from build123d import *

# Parameters (mm, degrees)
BOSS_EXTRUDE1_DEPTH = 4
BOSS_EXTRUDE1_DRAFT = 1
SHELL1_T            = -0.5
SKETCH2_R           = 2
BOSS_EXTRUDE2_DEPTH = 5.5
BOSS_EXTRUDE2_TAPER = 1.5
CIRPATTERN1_COUNT   = 4
SKETCH4_R           = 1.605977431
CUT_EXTRUDE1_DEPTH  = 5.5
CUT_EXTRUDE1_DRAFT  = 1.5
RIB2_START          = -8.069744096
RIB2_DEPTH          = 6.232014751
RIB2_START_2        = 1.837729345
RIB2_2_DEPTH        = 6.232014751
RIB2_START_3        = -0.25
RIB2_3_DEPTH        = 0.4999999
RIB2_START_4        = -5.909834066
RIB2_4_DEPTH        = 4.072104721
RIB2_5_DEPTH        = 4.072104621


with BuildPart() as part:
    # Sketch1 → Boss-Extrude1 (with draft: the straight prism first)
    with BuildSketch(Plane(origin=(0, 0, 0), x_dir=(1, 0, 0), z_dir=(0, 1, 0))):
        with BuildLine():
            Line((-7.5, -6.375), (7.5, -6.375))
            ThreePointArc((7.5, -6.375), (8.207106781, -6.082106781), (8.5, -5.375))
            Line((8.5, -5.375), (8.5, 5.375))
            ThreePointArc((8.5, 5.375), (8.207106781, 6.082106781), (7.5, 6.375))
            Line((7.5, 6.375), (-7.5, 6.375))
            ThreePointArc((-7.5, 6.375), (-8.207106781, 6.082106781), (-8.5, 5.375))
            Line((-8.5, 5.375), (-8.5, -5.375))
            ThreePointArc((-8.5, -5.375), (-8.207106781, -6.082106781), (-7.5, -6.375))
        make_face()
    extrude(amount=-BOSS_EXTRUDE1_DEPTH)
    # Boss-Extrude1: the draft: its side faces are tilted about the plane it starts from
    boss_extrude1_sides = [part.faces().sort_by_distance(p)[0] for p in [
        (0, -2, 6.375),
        (8.207106781, -2, 6.082106781),
        (8.5, -2, 0),
        (8.207106781, -2, -6.082106781),
        (0, -2, -6.375),
        (-8.207106781, -2, -6.082106781),
        (-8.5, -2, 0),
        (-8.207106781, -2, 6.082106781),
    ]]
    draft(boss_extrude1_sides, Plane(origin=(0, 0, 0), x_dir=(1, 0, 0), z_dir=(0, 1, 0)), BOSS_EXTRUDE1_DRAFT)

    # Shell1
    shell1_openings = [part.faces().sort_by_distance(p)[0] for p in [
        (0, -4, 0),
    ]]
    offset(amount=SHELL1_T, openings=shell1_openings, kind=Kind.INTERSECTION)

    # Sketch2 → Boss-Extrude2 (add)
    with BuildSketch(Plane.XZ.offset(0.5)):
        Circle(SKETCH2_R)
    extrude(amount=BOSS_EXTRUDE2_DEPTH, taper=BOSS_EXTRUDE2_TAPER)

    # Rib1: read off the stored shape, not the designer's step
    # Rib1: loft between two sections, ruled curve by curve
    rib1_from = [
        Edge.make_line((1.982302644, -0.5, 0.265473592), (2.872170331, -0.5, 0.25)),
        Edge.make_line((1.982302644, -0.5, -0.265473592), (2.872170331, -0.5, -0.25)),
        Edge.make_line((2.872170331, -0.5, -0.25), (2.872170331, -0.5, 0.25)),
        Edge.make_line((1.982302644, -0.5, -0.265473592), (1.982302644, -0.5, 0.265473592)),
    ]
    rib1_to = [
        Edge.make_line((1.837729445, -6, 0.259620323), (2.390982681, -6, 0.25)),
        Edge.make_line((1.837729445, -6, -0.259620323), (2.390982681, -6, -0.25)),
        Edge.make_line((2.390982681, -6, -0.25), (2.390982681, -6, 0.25)),
        Edge.make_line((1.837729445, -6, -0.259620323), (1.837729445, -6, 0.259620323)),
    ]
    rib1 = Solid(Shell([*[Face.make_surface_from_curves(rib1_from[k], rib1_to[k]) for k in range(4)], Face(Wire(rib1_from)), Face(Wire(rib1_to))]))
    add(rib1)

    # CirPattern1: Rib1 ×4 about axis
    cirpattern1_axis = Axis((0, 0, 0), (0, 1, 0))
    for i in range(1, CIRPATTERN1_COUNT):
        add(rib1.rotate(cirpattern1_axis, i * 360 / CIRPATTERN1_COUNT))


with BuildPart() as cut_extrude1_tool:
    # Sketch4 → Cut-Extrude1 (with draft: the straight prism first)
    with BuildSketch(Plane.XZ.offset(6)):
        Circle(SKETCH4_R)
    extrude(amount=-CUT_EXTRUDE1_DEPTH)
    # Cut-Extrude1: the draft: its side faces are tilted about the plane it starts from
    cut_extrude1_sides = [cut_extrude1_tool.faces().sort_by_distance(p)[0] for p in [
        (-1.605977431, -3.25, 0),
    ]]
    draft(cut_extrude1_sides, Plane.XZ.offset(6), CUT_EXTRUDE1_DRAFT)


with BuildPart() as part_1:
    add(part.part)

    # Cut-Extrude1: cut by cut_extrude1_tool
    add(cut_extrude1_tool.part, mode=Mode.SUBTRACT)

    # Sweep1: sweep along a path in Sketch6
    with BuildLine(Plane(origin=(0, -2, 0), x_dir=(1, 0, 0), z_dir=(0, 1, 0))) as sweep1_path:
        Line((8.56982026, -5.375), (8.56982026, 5.375))
        ThreePointArc((8.56982026, 5.375), (8.25647716, 6.13147716), (7.5, 6.44482026))
        Line((7.5, 6.44482026), (-7.5, 6.44482026))
        ThreePointArc((-7.5, 6.44482026), (-8.25647716, 6.13147716), (-8.56982026, 5.375))
        Line((-8.56982026, 5.375), (-8.56982026, -5.375))
        ThreePointArc((-8.56982026, -5.375), (-8.25647716, -6.13147716), (-7.5, -6.44482026))
        Line((-7.5, -6.44482026), (7.5, -6.44482026))
        ThreePointArc((7.5, -6.44482026), (8.25647716, -6.13147716), (8.56982026, -5.375))
    # Sketch5 → Sweep1 (sweep)
    with BuildSketch(Plane(origin=(0, 0, 0), x_dir=(0, 0, -1), z_dir=(1, 0, 0))):
        Polygon((-6.70991013, -2), (-6.44482026, -4), (-6.40991013, -2), align=None)
    sweep(path=sweep1_path.line)

    # Rib2: read off the stored shape, not the designer's step
    # Rib2 outline → Rib2 (add)
    with BuildSketch(Plane.YZ.offset(RIB2_START)):
        Polygon((-0.5, 0.276182597), (-2, 0.25), (-2, -0.25), (-0.5, -0.276182597), align=None)
    extrude(amount=RIB2_DEPTH)

    # Rib2 2 outline → Rib2 2 (add)
    with BuildSketch(Plane.YZ.offset(RIB2_START_2)):
        Polygon((-0.5, 0.276182597), (-2, 0.25), (-2, -0.25), (-0.5, -0.276182597), align=None)
    extrude(amount=RIB2_2_DEPTH)

    # Rib2 3 outline → Rib2 3 (add)
    with BuildSketch(Plane.YZ.offset(RIB2_START_3)):
        Polygon((-2, 2.740937336), (-0.5, 2.872170331), (-0.5, 5.883651368), (-2, 5.909833966), align=None)
        Polygon((-0.5, -5.883651368), (-0.5, -2.872170331), (-2, -2.740937336), (-2, -5.909833966), align=None)
    extrude(amount=RIB2_3_DEPTH)

    # Rib2 4 outline → Rib2 4 (add)
    with BuildSketch(Plane.XY.offset(RIB2_START_4)):
        Polygon((0.25, -2), (0.276182597, -0.5), (0.2499999, -0.5), align=None)
        Polygon((-0.276182597, -0.5), (-0.25, -2), (-0.25, -0.5), align=None)
    extrude(amount=RIB2_4_DEPTH)

    # Rib2 5 outline → Rib2 5 (add)
    with BuildSketch(Plane.XY.offset(RIB2_START_2)):
        Polygon((0.25, -2), (0.276182597, -0.5), (0.2499999, -0.5), align=None)
        Polygon((-0.276182597, -0.5), (-0.25, -2), (-0.25, -0.5), align=None)
    extrude(amount=RIB2_5_DEPTH)


solid = part_1.part
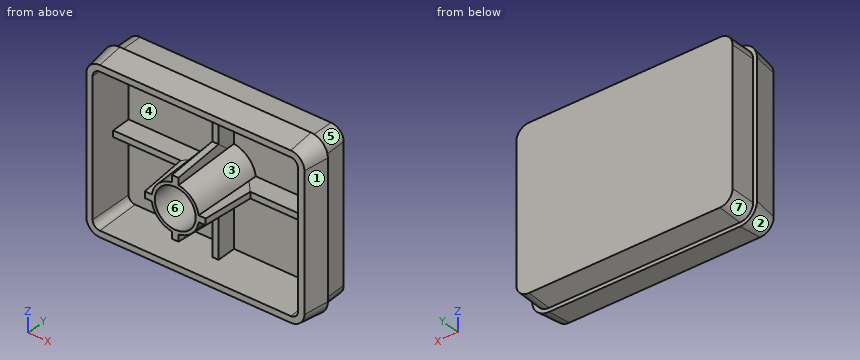
Geometry: final body of the model. Coordinates: model frame, mm. Face numbers are marked on the shaded views. A direction names the side the tool comes from. Round coordinates to 2 decimals unless told otherwise and drop trailing zeros. Loops run counter-clockwise (first coordinate to the right, second up) from the corner with the lowest first, then second, coordinate; pieces in that order, holes last.
Q1. Pull-direction query (Z, two-part tool) for the marked faces 1, 2 and 3; classes: released by +Z, released by -Z, zero draft, split by the parting line, or undercut.
Q2. Material intervals for L1, parallel to Z at x = -6, y = -1.75; L2, parallel to X at y = -0.75, z = 4.25; L3, parallel to Y at x = 4, z = -2.75, sorted ascending.
Q3. Section B-B on x = -4.25. Return loops of the section in (y, z) (3 decimals), plus the area to 3 significant figures.
Q4. Pin query (flat end, axial travel): P1, Ø8, axis at x = -1, z = 0, coming from the +Y side; P2, Ø1.5, axis at y = -4, z = 1, coming from the -X side; P3, Ø3, axis at x = -3, z = -4, coming from the -Y side; P4, Ø1.5, axis at x = -5, y = -3, coming from the +Z side. Return the tip coordinate at first contact, or that it passes through.
Q5. Access query for the marked faces 4, 5, 6 and 7. Directions: +Z, -Z, +X, -X, +Y, -Y. A direction counts if a zero-diameter tool reaches every point of the face in a straight line with its end or side. Return the directions, or none.
Q6. Section C-C on y = -3.5. State how many separate pieces and enclosed holes the cut face has, plus the area to 3 significant figures.
Q7. Section A-A on z = -3.5. Return loops of the section in (x, y), plus the area to 3 significant figures.
Evaluation:
1. face 1: zero draft
1. face 2: released by -Z
1. face 3: undercut
2. L1: z = -6.41 to -5.91, -0.25 to 0.25, 5.91 to 6.41
2. L2: x = -8.51 to -8.01, -0.27 to 0.27, 8.01 to 8.51
2. L3: y = -0.5 to 0
3. outline: (-4, -6.445) - (-2, -6.71) - (-2, -6.41) - (0, -6.375) - (0, 6.375) - (-2, 6.41) - (-2, 6.71) - (-4, 6.445) - (-4, 5.945) - (-0.5, 5.884) - (-0.5, 0.276) - (-2, 0.25) - (-2, -0.25) - (-0.5, -0.276) - (-0.5, -5.884) - (-4, -5.945) - close
3. area: 11.3 mm2
4. P1: stops at y = 0
4. P2: stops at x = -8.67
4. P3: stops at y = -0.5
4. P4: stops at z = 6.68
5. face 4: -Y
5. face 5: +Z, +X, +Y
5. face 6: none
5. face 7: -Z, -X, +Y
6. separate pieces: 2
6. enclosed holes: 2
6. area: 36.9 mm2
7. outline: (-8.83, -2) - (-8.57, -4) - (-8.07, -4) - (-8.01, -0.5) - (-0.28, -0.5) - (-0.25, -2) - (0.25, -2) - (0.28, -0.5) - (8.01, -0.5) - (8.07, -4) - (8.57, -4) - (8.83, -2) - (8.53, -2) - (8.5, 0) - (-8.5, 0) - (-8.53, -2) - close
7. area: 13.4 mm2
